Input: part model. Units: mm. Frame: model coordinates. A direction names the side the tool comes from. Give positions to 0.01 mm unless a question says otherwise; leave off trailing zeros. Loops run counter-clockwise (first coordinate to the right, second up) from the corner with the lowest first, then second, coordinate; pieces in that order, holes last. Notation, with made-up numbers: M -1.75,25.25 L 50.25,25.25 A23 cw 50.25,52.25 Z; hole C 59,30.25 d10. An arc over 180 degrees is marked long. Answer as a JSON object with one key per item and string values. Group by question number.
1) Section query C-C on x = 2.75. Return loops of the section in (y, z), plus the area to 3 significant figures.
2) Draft query along Y for faces 1 (the cylindrical face through (-1.227, -5.847, 0.077)), 2 (the cylindrical face through (3.23, 6.21, -9.3)), 3 (the cylindrical face through (-5.94, -0.64, 0.08)). Return one class per face: +Y half, -Y half, draft (parallel to the pull), parting line (faces both ways), or undercut.
3) Ray query, L1, parallel to Y at x = 0, z = 2; L2, parallel to Z at x = 3.75, y = -5; L3, parallel to Z at x = -1.75, y = -6.5. Return the intervals inside material, ascending.
4) Section query B-B on z = -10.25. Return loops of the section in (x, y), plus the area to 3 significant figures.
5) Access query for faces 4 (the flat face through (3, -3, 6.5)), 5 (the cylindrical face through (1.26, -5.84, 0.08)), 6 (the flat face through (6, 2, -5.5)), 7 (the cylindrical face through (5.943, -0.609, 0.077)). Directions: +Z, -Z, +X, -X, +Y, -Y. A direction counts if a zero-diameter tool reaches every point of the face in a straight line with its end or side. Return the directions, or none.
6) First-contact query: P1, Ø5, axis at y = 0, z = 3.5, coming from the +X side; P2, Ø3.5, axis at y = 0, z = -9.25, coming from the +X side; P3, Ø1.5, axis at x = 2, y = 2.5, coming from the +Z side. Flat tips, straight axial feed; report the tip coordinate or a pass-through.
7) Section query D-D on y = 1.75. Return loops of the section in (x, z).
8) Section query A-A on x = 0. Return loops of the section in (y, z), plus the area to 3 significant figures.
from build123d import *

# Parameters (mm, degrees)
SKETCH1_R           = 6.843972439
BOSS_EXTRUDE1_DEPTH = 5.5
CUT_EXTRUDE1_DEPTH  = 15.65195951
CIRPATTERN1_COUNT   = 15
SKETCH3_R           = 7
BOSS_EXTRUDE2_DEPTH = 1
BOSS_EXTRUDE3_START = 7.5
SKETCH4_R           = 7
BOSS_EXTRUDE3_DEPTH = 7.5
SKETCH5_R           = 4
CUT_EXTRUDE2_DEPTH  = 22.868927729
SKETCH6_R           = 2
CUT_EXTRUDE3_DEPTH  = 17.340134638
CIRPATTERN2_COUNT   = 2
CIRPATTERN2_ANGLE   = 90


with BuildPart() as part:
    # Sketch1 → Boss-Extrude1 (new, symmetric)
    with BuildSketch(Plane.XY):
        Circle(SKETCH1_R)
    extrude(amount=BOSS_EXTRUDE1_DEPTH, both=True)

    # Sketch2 → Cut-Extrude1 (cut, through all)
    with BuildSketch(Plane.XY.offset(5.5)):
        with BuildLine():
            ThreePointArc((-1.117417151, 6.752135785), (-0.9397987, 6.71772722), (-0.827629371, 6.57577545))
            ThreePointArc((-0.827629371, 6.57577545), (0, 5.973972439), (0.827629371, 6.57577545))
            ThreePointArc((0.827629371, 6.57577545), (0.9397987, 6.71772722), (1.117417151, 6.752135785))
            ThreePointArc((1.117417151, 6.752135785), (0, 6.843972439), (-1.117417151, 6.752135785))
        make_face()
    cut_extrude1 = extrude(amount=-CUT_EXTRUDE1_DEPTH, mode=Mode.SUBTRACT)

    # CirPattern1: Cut-Extrude1 ×15 about axis
    cirpattern1_axis = Axis((0, 0, 0), (0, 0, 1))
    for i in range(1, CIRPATTERN1_COUNT):
        add(cut_extrude1.rotate(cirpattern1_axis, i * 360 / CIRPATTERN1_COUNT), mode=Mode.SUBTRACT)

    # Sketch3 → Boss-Extrude2 (add)
    with BuildSketch(Plane.XY.offset(5.5)):
        Circle(SKETCH3_R)
    extrude(amount=BOSS_EXTRUDE2_DEPTH)

    # Sketch4 → Boss-Extrude3 (add)
    with BuildSketch(Plane(origin=(0, 0, -5.5), x_dir=(-1, 0, 0), z_dir=(0, 0, -1)).offset(BOSS_EXTRUDE3_START)):
        with Locations(Location((0, 0, 0), (0, 0, 180))):
            Circle(SKETCH4_R)
    extrude(amount=-BOSS_EXTRUDE3_DEPTH)

    # Sketch5 → Cut-Extrude2 (cut, through all)
    with BuildSketch(Plane.XY.offset(6.5)):
        Circle(SKETCH5_R)
    extrude(amount=-CUT_EXTRUDE2_DEPTH, mode=Mode.SUBTRACT)

    # Sketch6 → Cut-Extrude3 (cut, through all)
    with BuildSketch(Plane(origin=(0, 0, 0), x_dir=(0, 0, -1), z_dir=(1, 0, 0))):
        with Locations(Location((9.25, 0, 0), (0, 0, 180))):
            Circle(SKETCH6_R)
    cut_extrude3 = extrude(amount=CUT_EXTRUDE3_DEPTH, mode=Mode.SUBTRACT)

    # CirPattern2: Cut-Extrude3 ×2 about axis
    cirpattern2_axis = Axis((0, 0, -13), (0, 0, -1))
    for i in range(1, CIRPATTERN2_COUNT):
        add(cut_extrude3.rotate(cirpattern2_axis, i * CIRPATTERN2_ANGLE / (CIRPATTERN2_COUNT - 1)), mode=Mode.SUBTRACT)


solid = part.part
Output:
{
 "1": {"outline": "M -6.44,-13 L -2.9,-13 L -2.9,6.5 L -6.44,6.5 L -6.44,5.5 L -6.27,5.5 L -6.27,-5.5 L -6.44,-5.5 Z; M 2.9,-13 L 6.44,-13 L 6.44,-5.5 L 5.38,-5.5 L 5.38,5.5 L 6.44,5.5 L 6.44,6.5 L 2.9,6.5 Z", "area": "124 mm^2"},
 "2": {"face 1": "-Y half", "face 2": "parting line", "face 3": "undercut"},
 "3": {"L1": "y = -6.84 to -4, 4 to 5.97", "L2": "z = -13 to -5.5, 5.5 to 6.5", "L3": "z = -13 to -10.22, -8.28 to -5.5, 5.5 to 6.5"},
 "4": {"outline": "M -1.73,-6.78 L -1.73,-3.61 A4 cw long 3.61,1.73 L 6.78,1.73 A7 ccw long Z; M 1.73,-6.78 A7 ccw 6.78,-1.73 L 3.61,-1.73 A4 cw 1.73,-3.61 Z", "area": "82.5 mm^2"},
 "5": {"face 4": "+Z, +X, -X, +Y, -Y", "face 5": "-Y", "face 6": "none", "face 7": "+X"},
 "6": {"P1": "stops at x = 7", "P2": "stops at x = -3.6", "P3": "passes through"},
 "7": {"outline": "M -6.78,-13 L -3.6,-13 L -3.6,6.5 L -6.78,6.5 L -6.78,5.5 L -5.72,5.5 L -5.72,-5.5 L -6.78,-5.5 Z; M 3.6,-13 L 6.78,-13 L 6.78,-10.22 L 3.6,-10.22 Z; M 3.6,-8.28 L 6.78,-8.28 L 6.78,-5.5 L 5.72,-5.5 L 5.72,5.5 L 6.78,5.5 L 6.78,6.5 L 3.6,6.5 Z"},
 "8": {"outline": "M -7,-13 L -4,-13 L -4,-11.25 L -7,-11.25 Z; M -7,-7.25 L -4,-7.25 L -4,6.5 L -7,6.5 L -7,5.5 L -6.84,5.5 L -6.84,-5.5 L -7,-5.5 Z; M 4,-13 L 7,-13 L 7,-5.5 L 5.97,-5.5 L 5.97,5.5 L 7,5.5 L 7,6.5 L 4,6.5 Z", "area": "92.0 mm^2"}
}
